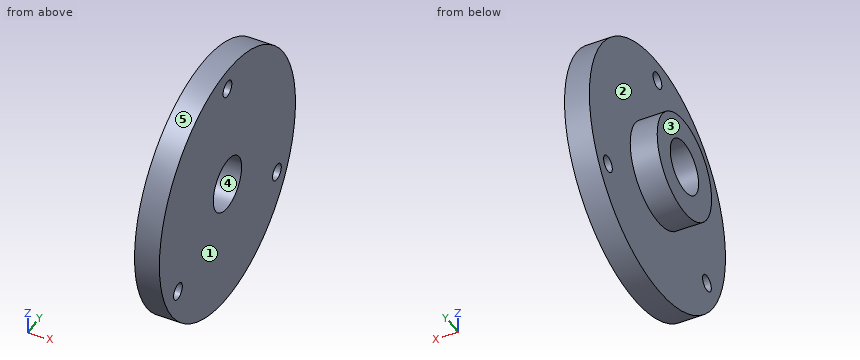
Autodesk Inventor part; units mm, degrees
ref_plane "YZ Plane" through (0, 0, 0) normal (1, 0, 0) x (0, 1, 0)
ref_plane "XZ Plane" through (0, 0, 0) normal (0, 1, 0) x (-1, 0, 0)
ref_plane "XY Plane" through (0, 0, 0) normal (0, 0, 1) x (1, 0, 0)
sketch "Sketch1" plane through (0, 0, 0) normal (1, 0, 0) x (0, 1, 0)
  circle A0 centre (0, 0) radius 62.5
  circle A1 centre (0, 0) radius 25
  circle A2 centre (0, 0) radius 13
  circle A3 centre (0, 0) radius 52.5 construction
  circle A4 centre (0, 52.5) radius 4
  circle A5 centre (-45.4663, -26.25) radius 4
  circle A6 centre (45.4663, -26.25) radius 4
  dimension "d0" = 50
  dimension "d1" = 26
  dimension "d2" = 125
  dimension "d7" = 8
  dimension "d8" = 10
  dimension "d11" = 360
extrude "Extrusion1" add sketch "Sketch1" along normal blind 12 contours A0 | A1 | A4 | A5 | A6
extrude "Extrusion2" add sketch "Sketch1" against normal blind 13 contours A1
extrude "Extrusion3" cut sketch "Sketch1" along normal blind 45.5 contours A4 | A5 | A6
properties part number "Chuck Backplate"
Geometry check sheet. Reference: the model listing, model coordinates, mm. Face numbers are marked on the shaded views. A direction names the side the tool comes from. Coordinates: 2 decimals unless noted, no trailing zeros. Order: outer loops, then holes, each group sorted by start corner. A loop starts at its lowest first (then second) coordinate and runs counter-clockwise, first axis right, second up.
Item 1: Section check D-D (x = -9.75). Enter the section's corners in (y, z), plus the area to 3 significant figures.
Item 2: Scan lines: line 1 along Z through (x, y) = (3.75, 0); line 2 along Y through (x, z) = (7.5, -26.25); line 3 along Z through (x, y) = (-7.25, 0). Record each from-to range of solid material in increasing order.
Item 3: Tool access check on the marked faces 1 and 2. Record the directions out of +Z, -Z, +X, -X, +Y, -Y that give a thin tool (end or side, any length) a straight path to the whole face; none if there is none.
Item 4: Section check B-B (x = 5.75). Enter the section's corners in (y, z), plus the area to 3 significant figures.
Item 5: Mould release check, pull along Y, two halves, no side actions. Record for the marked faces 3, 4 and 5: released by +Y, released by -Y, zero draft, split by the parting line, or undercut.
Item 6: Depth check by flat-ended pin: pin 1 (2 mm diameter, centred on x = 6.5, z = -3, fed in from +Y); pin 2 (8 mm diameter, centred on x = -2, y = 30, fed in from -Z); pin 3 (1 mm diameter, centred on y = -42, z = -14.5, fed in from -X). Enter the tip coordinate at first touch or a pass-through.
Item 7: Section check C-C (y = 0). Enter the section's corners in (x, z).
Item 8: Section check A-A (z = 0). Enter the section's corners in (x, y).
Check sheet entries:
1. outline: circle Ø50 at (0, 0); hole circle Ø26 at (0, 0)
1. area: 1,430 mm2
2. line 1: z = -62.5 to -13, 13 to 48.5, 56.5 to 62.5
2. line 2: y = -56.72 to -49.47, -41.47 to 41.47, 49.47 to 56.72
2. line 3: z = -25 to -13, 13 to 25
3. face 1: +Z, -Z, +X, +Y, -Y
3. face 2: -X
4. outline: circle Ø125 at (0, 0); hole circle Ø8 at (-45.47, -26.25); hole circle Ø26 at (0, 0); hole circle Ø8 at (0, 52.5); hole circle Ø8 at (45.47, -26.25)
4. area: 11,600 mm2
5. face 3: zero draft
5. face 4: undercut
5. face 5: split by the parting line
6. pin 1: stops at y = 62.47
6. pin 2: stops at z = -56.59
6. pin 3: stops at x = 0
7. outline: (-13, -25) - (0, -25) - (0, -62.5) - (12, -62.5) - (12, -13) - (-13, -13) - close; (-13, 13) - (12, 13) - (12, 48.5) - (0, 48.5) - (0, 25) - (-13, 25) - close; (0, 56.5) - (12, 56.5) - (12, 62.5) - (0, 62.5) - close
8. outline: (-13, -25) - (0, -25) - (0, -62.5) - (12, -62.5) - (12, -13) - (-13, -13) - close; (-13, 13) - (12, 13) - (12, 62.5) - (0, 62.5) - (0, 25) - (-13, 25) - close
